from build123d import *

# Parameters (mm, degrees)
F0_W     = 101.6
F0_H     = 25.8370920686
F1_DEPTH = 25.4
F3_DEPTH = 25.4
F2_R     = 8.8764145502
F4_DEPTH = 25.4
F5_DEPTH = 25.4


with BuildPart() as f1:
    # F0 (on Top) → F1 (new body)
    with BuildSketch(Plane.XY):
        Rectangle(F0_W, F0_H)
    extrude(amount=F1_DEPTH)

    # F3 (add): a face of the model
    f3_faces = [f1.faces().sort_by_distance(p)[0] for p in [
        (-50.8, 0, 12.7),
    ]]
    extrude(f3_faces, amount=F3_DEPTH)

    # F2 (on face) → F4 (join)
    with BuildSketch(Plane.YZ.offset(50.8)):
        with Locations((0, 12.3842312023)):
            Circle(F2_R)
    extrude(amount=F4_DEPTH)

    # F5 (add): a face of the model
    f5_faces = [f1.faces().sort_by_distance(p)[0] for p in [
        (76.2, 0, 12.3842312023),
    ]]
    extrude(f5_faces, amount=F5_DEPTH)


solid = f1.part
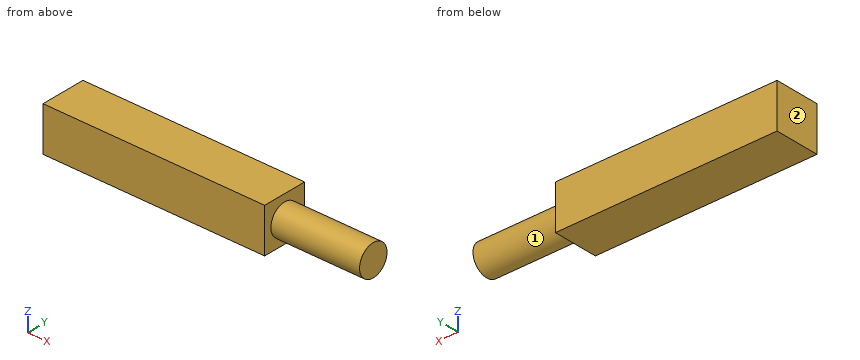
Source: CAD feature listing. Evaluate the final solid. Frame: model axes, mm. Face numbers are marked on the shaded views. A direction names the side the tool comes from. Give positions to 0.01 mm unless a question says otherwise; leave off trailing zeros. Loops run counter-clockwise (first coordinate to the right, second up) from the corner with the lowest first, then second, coordinate; pieces in that order, holes last. Notation, with made-up numbers: (87, -26.5) -> (127, -26.5) arc R12 ccw to (127, -6.5) -> close; hole circle Ø7 at (6, 5.5). An arc over 180 degrees is marked (long way). Use a Markdown table: item, result. Add a question column.
1) First-contact query: pin 1 (6 mm diameter, centred on x = 56, y = 3, fed in from +Z); pin 2 (3 mm diameter, centred on x = 24, y = -7, fed in from -Z). Flat tips, straight axial feed; report the tip coordinate or a pass-through.
2) Section query A-A, the plane y = 0. Return the cut outline in (x, z).
3) Section query B-B, the plane z = 19. Return the cut outline in (x, y), then the cut area to 3 significant figures.
4) Reachability of the marked faces 1 and 2 from +Z, -Z, +X, -X, +Y, -Y: full face, straight path, thin tool, end or side. Return the list, or none.
5) Line query: line 1 along X through (y, z) = (-8, 22); line 2 along Z through (x, y) = (64, -1.5); line 3 along Z through (x, y) = (64, 2.75). Output: solid intervals per line, ascending. Write a range as [from, to].
6) Section query C-C, the plane z = 1.75. Return the cut outline in (x, y), then the cut area to 3 significant figures.
Numbers:
| question | item | result |
|---|---|---|
| 1 | pin 1 | stops at z = 21.26 |
| 1 | pin 2 | stops at z = 0 |
| 2 | outline | (-76.2, 0) -> (50.8, 0) -> (50.8, 3.51) -> (101.6, 3.51) -> (101.6, 21.26) -> (50.8, 21.26) -> (50.8, 25.4) -> (-76.2, 25.4) -> close |
| 3 | outline | (-76.2, -12.92) -> (50.8, -12.92) -> (50.8, -5.92) -> (101.6, -5.92) -> (101.6, 5.92) -> (50.8, 5.92) -> (50.8, 12.92) -> (-76.2, 12.92) -> close |
| 3 | area | 3,880 mm2 |
| 4 | face 1 | +X |
| 4 | face 2 | +Z, -Z, -X, +Y, -Y |
| 5 | line 1 | x = [-76.2, 50.8] |
| 5 | line 2 | z = [3.64, 21.13] |
| 5 | line 3 | z = [3.94, 20.82] |
| 6 | outline | (-76.2, -12.92) -> (50.8, -12.92) -> (50.8, 12.92) -> (-76.2, 12.92) -> close |
| 6 | area | 3,280 mm2 |
